from build123d import *

# Parameters (mm, degrees)
BASPROSKE_W                              = 28
BASPROSKE_H                              = 28.5
TOOTHCUT_DEPTH                           = 50.076470941
TEETHCUTS_COUNT                          = 17
TEETHCUTS_ANGLE                          = 338.823529412
BORSKE_R                                 = 0.4
BORE_DEPTH                               = 50.0000508
CUT_EXTRUDE1_DEPTH                       = 21
CBORE_FOR_M3_PAN_HEAD_SCREW1_D           = 2.8
CBORE_FOR_M3_PAN_HEAD_SCREW1_CBORE_D     = 7
CBORE_FOR_M3_PAN_HEAD_SCREW1_CBORE_DEPTH = 2.4
FILLET1_R                                = 0.5


with BuildPart() as part:
    # BasProSke → Base-Revolve (revolve)
    with BuildSketch(Plane(origin=(0, 0, 0), x_dir=(1, 0, 0), z_dir=(0, 1, 0)), mode=Mode.PRIVATE) as base_revolve_sk:
        with Locations((14, 14.25)):
            Rectangle(BASPROSKE_W, BASPROSKE_H)
    revolve(base_revolve_sk.sketch.rotate(Axis((-10, 0, 0), (1, 0, 0)), 180), axis=Axis((-10, 0, 0), (1, 0, 0)))

    # TooCutSke → ToothCut (cut, through all)
    with BuildSketch(Plane(origin=(0, 0, 0), x_dir=(0, 0, -1), z_dir=(1, 0, 0))):
        with BuildLine():
            ThreePointArc((1.540279816, 21.694389576), (0, 21.749), (-1.540279816, 21.694389576))
            ThreePointArc((-1.540279816, 21.694389576), (-2.457007956, 25.198716871), (-4.540621854, 28.161697363))
            ThreePointArc((-4.540621854, 28.161697363), (0, 28.5254), (4.540621854, 28.161697363))
            ThreePointArc((4.540621854, 28.161697363), (2.457007956, 25.198716871), (1.540279816, 21.694389576))
        make_face()
    toothcut = extrude(amount=TOOTHCUT_DEPTH, mode=Mode.SUBTRACT)

    # TeethCuts: ToothCut ×17 about axis
    teethcuts_axis = Axis((-10, 0, 0), (1, 0, 0))
    for i in range(1, TEETHCUTS_COUNT):
        add(toothcut.rotate(teethcuts_axis, i * TEETHCUTS_ANGLE / (TEETHCUTS_COUNT - 1)), mode=Mode.SUBTRACT)

    # BorSke → Bore (cut, symmetric)
    with BuildSketch(Plane(origin=(0, 0, 0), x_dir=(0, 0, -1), z_dir=(1, 0, 0))):
        with Locations(Location((0, 0, 0), (0, 0, 180))):
            Circle(BORSKE_R)
    extrude(amount=BORE_DEPTH, both=True, mode=Mode.SUBTRACT)

    # Sketch1 → Cut-Extrude1 (cut)
    with BuildSketch(Plane.ZY):
        Polygon((0, -7.5), (6.495190528, -3.75), (6.495190528, 3.75), (0, 7.5), (-6.495190528, 3.75), (-6.495190528, -3.75), align=None)
    extrude(amount=-CUT_EXTRUDE1_DEPTH, mode=Mode.SUBTRACT)

    # CBORE for M3 Pan Head Screw1 (through all)
    with Locations(Plane(origin=(28, 0, 0), x_dir=(0, 0, -1), z_dir=(1, 0, 0))):
        with Locations((0, 0)):
            CounterBoreHole(CBORE_FOR_M3_PAN_HEAD_SCREW1_D / 2, CBORE_FOR_M3_PAN_HEAD_SCREW1_CBORE_D / 2, CBORE_FOR_M3_PAN_HEAD_SCREW1_CBORE_DEPTH)

    # Fillet1
    fillet1_edges = [part.edges().sort_by_distance(p)[0] for p in [
        (10.5, -7.5, 0),
        (10.5, -3.75, -6.495190528),
        (10.5, 3.75, -6.495190528),
        (10.5, 7.5, 0),
        (10.5, 3.75, 6.495190528),
        (10.5, -3.75, 6.495190528),
        (0, -5.625, -3.247595264),
        (0, -5.625, 3.247595264),
        (0, 0, 6.495190528),
        (0, 5.625, 3.247595264),
        (0, 5.625, -3.247595264),
        (0, 0, -6.495190528),
    ]]
    fillet(fillet1_edges, radius=FILLET1_R)


solid = part.part
Verification items for the finished model (mm, model axes). A direction names the side the tool comes from. Give positions to 0.01 mm unless a question says otherwise; leave off trailing zeros. Order: outer loops, then holes, each group sorted by start corner. A loop starts at its lowest first (then second) coordinate and runs counter-clockwise, first axis right, second up. Notation, with made-up numbers: M 25,59 L 82,59 A31 ccw 82,97 Z; hole C 81.25,-11 d7. An arc over 180 degrees is marked long. Answer as a JSON object with one key per item and string values. Group by question number.
1) Cross-section at A-A (y = -23.5). Enter the section's corners in (x, z), then the cut area to 3 significant figures.
2) Scan lines: line 1 along Y through (x, z) = (23.75, 0); line 2 along Y through (x, z) = (13.25, -22.5); line 3 along Y through (x, z) = (24.5, 23.5). Record each from-to range of solid material in increasing order. Write a range as [from, to].
3) Mould release check, pull along Y, two halves, no side actions. Record for faces 4 (the face through (13.804, 9.034, -23.687)), 5 (the face through (13.8, 25.23, -2.47)), 6 (the face through (14.196, -26.579, -10.286)): released by +Y, released by -Y, zero draft, split by the parting line, or undercut.
4) Depth check by flat-ended pin: pin 1 Ø6 at (x, z) = (15, -5.5) entering from -Y; pin 2 Ø2 at (x, z) = (5.5, 11.5) entering from -Y; pin 3 Ø8 at (x, y) = (23, 21.5) entering from +Z; pin 4 Ø2.5 at (y, z) = (0, 0) entering from -X. Enter the tip coordinate at first touch or a pass-through.
5) Access from +Z, -Z, +X, -X, +Y, -Y to the whole of each face (thin tool, end or side, straight path). Record for faces 1 (the face through (26.817, -1.341, -3.233)), 2 (the face through (13.804, 4.789, 24.895)), 3 (the face through (10.61, 5.6, 3.29)).
6) Cross-section at B-B (y = 23). Enter the section's corners in (x, z), then the cut area to 3 significant figures.
Result sheet:
{
 "1": {"outline": "M 0,-11.24 L 28,-11.24 L 28,-6.52 L 0,-6.52 Z; M 0,-2.5 L 28,-2.5 L 28,2.5 L 0,2.5 Z; M 0,6.52 L 28,6.52 L 28,11.24 L 0,11.24 Z", "area": "404 mm2"},
 "2": {"line 1": "y = [-28.5, -1.4], [1.4, 21.75]", "line 2": "y = [-13.38, -8.46], [-4.63, 0.45], [3.77, 8.94], [15.01, 17.49]", "line 3": "y = [-13.45, -9.2], [-4.66, 0.34], [4.11, 9.03]"},
 "3": {"face 4": "undercut", "face 5": "released by +Y", "face 6": "released by -Y"},
 "4": {"pin 1": "stops at y = -25.95", "pin 2": "stops at y = -26.5", "pin 3": "stops at z = 22.49", "pin 4": "passes through"},
 "5": {"face 1": "+X", "face 2": "+Z, +X, -X", "face 3": "-X"},
 "6": {"outline": "M 0,-15.63 L 28,-15.63 L 28,-11.82 L 0,-11.82 Z; M 0,-6.81 L 28,-6.81 L 28,-1.73 L 0,-1.73 Z; M 0,1.73 L 28,1.73 L 28,6.81 L 0,6.81 Z; M 0,11.82 L 28,11.82 L 28,15.63 L 0,15.63 Z", "area": "497 mm2"}
}
